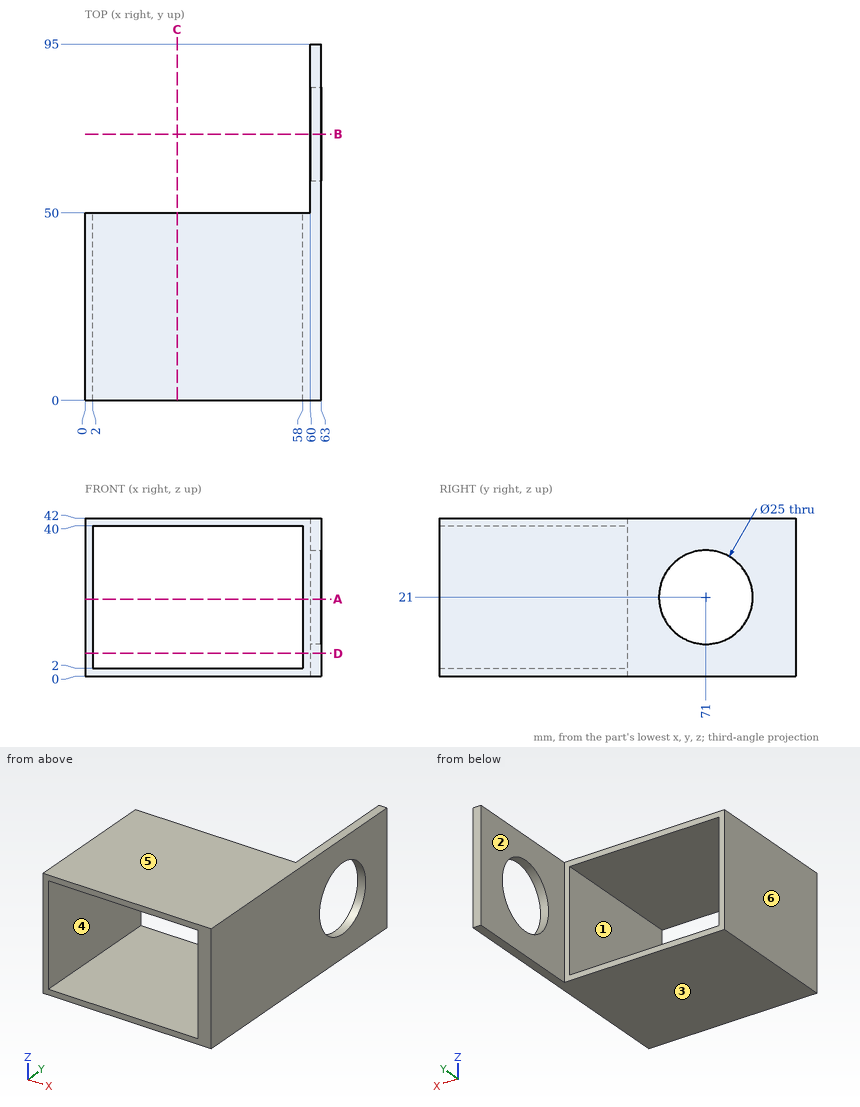
Design review of the part shown in the three views and the two pictorial views. Dimensions are in mm from the part's minimum x, y and z. A direction names the side the tool comes from. Give positions to 0.01 mm unless a question says otherwise; leave off trailing zeros. Write each loop counter-clockwise with the first axis right and the second up, starting at its lowest first coordinate (ties: lowest second). Pieces come first, ordered by that corner, then holes. Notation, with made-up numbers: M 79.5,32 L 97.5,32 A7 ccw 97.5,36 Z; hole C 42,-35 d8. An arc over 180 degrees is marked long. Answer as CSV lines item,"result".
1. Consider section C-C, the plane x = 24.5. Write out the cut boundary in (y, z).
Findings:
outline,"M 0,0 L 50,0 L 50,2 L 0,2 Z; M 0,40 L 50,40 L 50,42 L 0,42 Z"
2. For the marked faces 1, 2 and 3, list the 3-axis set-ups (+Z, -Z, +X, -X, +Y, -Y) from which the entire face can be reached by the end or side of a thin tool; tool diameter is ignored.
Findings:
face 1,"+Y, -Y"
face 2,"+Z, -Z, -X, +Y"
face 3,"-Z, +X, -X, +Y, -Y"
3. Wall thickness on line 1 (Z direction, x = 4, y = 18); line 2 (Y direction, x = 62, z = 21); line 3 (X direction, y = 30.5, z = 6.5): over which ranges is each line inside the solid? List them lowest first.
Findings:
line 1,"z = 0 to 2, 40 to 42"
line 2,"y = 0 to 58.5, 83.5 to 95"
line 3,"x = 0 to 2, 58 to 63"
4. Consider section B-B, the plane y = 71. Write out the cut boundary in (x, z), then the cut area to 3 significant figures.
Findings:
outline,"M 60,0 L 63,0 L 63,8.5 L 60,8.5 Z; M 60,33.5 L 63,33.5 L 63,42 L 60,42 Z"
area,"51.0 mm2"
5. For pin 1 (12.5 mm diameter, centred on y = 66.5, z = 11, fed in from -X), flat-tipped, find the tip position at first contact; note if it passes through.
Findings:
pin 1,"stops at x = 60"
6. Consider section A-A, the plane z = 20.5. Write out the cut boundary in (x, y).
Findings:
outline,"M 0,0 L 2,0 L 2,50 L 0,50 Z; M 58,0 L 63,0 L 63,58.51 L 60,58.51 L 60,50 L 58,50 Z; M 60,83.49 L 63,83.49 L 63,95 L 60,95 Z"
7. Draft analysis for pull direction Z (two halves, no side actions). For the marked faces 4, 5 and 6, state which applies: +Z half, -Z half, draft (parallel to the pull), parting line (faces both ways), or undercut.
Findings:
face 4,"undercut"
face 5,"+Z half"
face 6,"draft"
8. Consider section D-D, the plane z = 6. Write out the cut boundary in (x, y), then the cut area to 3 significant figures.
Findings:
outline,"M 0,0 L 2,0 L 2,50 L 0,50 Z; M 58,0 L 63,0 L 63,95 L 60,95 L 60,50 L 58,50 Z"
area,"485 mm2"
